Can you work these out from the drawing? Everything is in mm from the part's minimum corner. A direction names the side the tool comes from. Coordinates: 2 decimals unless noted, no trailing zeros. Order: outer loops, then holes, each group sorted by start corner. A loop starts at its lowest first (then second) coordinate and runs counter-clockwise, first axis right, second up. Notation, with made-up numbers: (75.5, 61) -> (110.5, 61) arc R23 ccw to (110.5, 81) -> close; hole circle Ø8 at (19, 66). An arc over 180 degrees is marked (long way). Use a Markdown table: item, result. Add a question column.
1) If we section it at C-C (z = 1.75): Write out the boundary of the cut face in (x, y), plus the area to 3 significant figures.
2) If I drill on L1, parallel to Y at x = 0.4, z = 8.5; L2, parallel to X at y = 2, z = 7.75; L3, parallel to Z at x = 2.75, y = 3.95, over which ranges is the centre line in solid material (lowest first)? Write a range as [from, to].
3) If we section it at B-B (y = 3.4): Write out the boundary of the cut face in (x, z).
4) Which directions (+Z, -Z, +X, -X, +Y, -Y) give clear straight access to the entire face, cutting with the end or side of a thin tool? Please do the marked faces 1, 2, 3 and 4.
5) If we section it at A-A (x = 3): Write out the boundary of the cut face in (y, z), plus the area to 3 significant figures.
6) Will these pins go through, and if not, where does the flat tip stop? pin 1 Ø1.5 at (x, y) = (1, 3) entering from -Z; pin 2 Ø2.5 at (x, y) = (2, 3) entering from +Z; pin 3 Ø2.5 at (x, z) = (1.5, 4.5) entering from +Y.
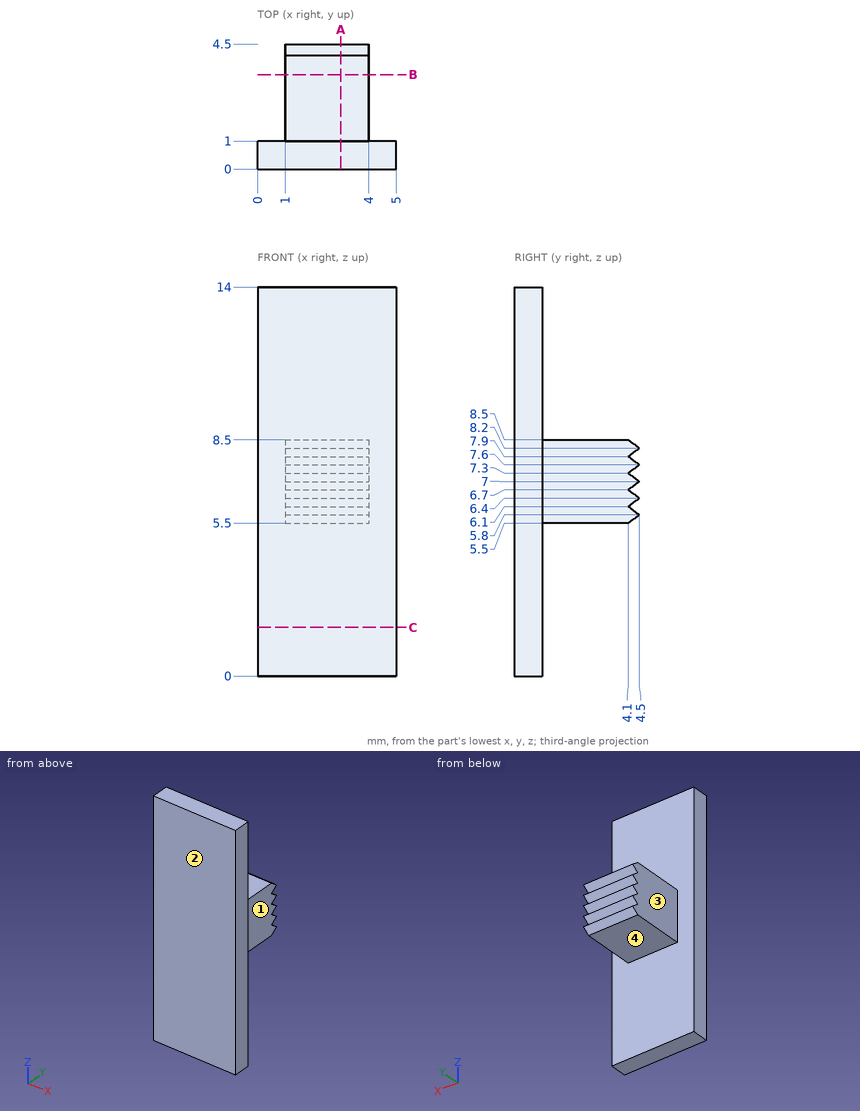
Answer sheet:
| question | item | result |
|---|---|---|
| 1 | outline | (0, 0) -> (5, 0) -> (5, 1) -> (0, 1) -> close |
| 1 | area | 5.00 mm2 |
| 2 | L1 | [0, 1] |
| 2 | L2 | [1, 4] |
| 2 | L3 | [5.5, 8.5] |
| 3 | outline | (1, 5.5) -> (4, 5.5) -> (4, 8.5) -> (1, 8.5) -> close |
| 4 | face 1 | +Z, -Z, +X, +Y |
| 4 | face 2 | +Z, -Z, +X, -X, -Y |
| 4 | face 3 | +Z, -Z, -X, +Y |
| 4 | face 4 | -Z, +X, -X, +Y |
| 5 | outline | (0, 0) -> (1, 0) -> (1, 5.5) -> (4.1, 5.5) -> (4.5, 5.8) -> (4.1, 6.1) -> (4.5, 6.4) -> (4.1, 6.7) -> (4.5, 7) -> (4.1, 7.3) -> (4.5, 7.6) -> (4.1, 7.9) -> (4.5, 8.2) -> (4.1, 8.5) -> (1, 8.5) -> (1, 14) -> (0, 14) -> close |
| 5 | area | 23.9 mm2 |
| 6 | pin 1 | z = 5.5 |
| 6 | pin 2 | z = 8.5 |
| 6 | pin 3 | y = 4.43 |
